Work out the finished part from the listing and answer in its coordinate system (mm). Give positions to 0.01 mm unless a question says otherwise; leave off trailing zeros. Write each loop counter-clockwise with the first axis right and the second up, starting at its lowest first coordinate (ties: lowest second). Pieces come first, ordered by that corner, then holes. Notation, with made-up numbers: (-27.75, 20.25) - (28.25, 20.25) arc R22 ccw to (28.25, 49.25) - close; hole circle Ø6 at (-12.5, -9). An arc over 180 degrees is marked (long way). Write item = value, one per line.
from build123d import *

# Parameters (mm, degrees)
ESBO_O1_R                = 3
RESSALTO_EXTRUS_O1_DEPTH = 5
FILETE1_R                = 6
RESSALTO_EXTRUS_O2_START = 5
RESSALTO_EXTRUS_O2_DEPTH = 5


with BuildPart() as part:
    # Esboço1 → Ressalto-extrusão1 (new body)
    with BuildSketch(Plane.XY):
        Polygon((-8, -8), (-8, 8), (0, 8), (42.879830598, -10.223928004), (37.120169402, -23.776071996), (0, -8), align=None)
        Circle(ESBO_O1_R, mode=Mode.SUBTRACT)
    extrude(amount=RESSALTO_EXTRUS_O1_DEPTH)

    # Filete1
    filete1_edges = [part.edges().sort_by_distance(p)[0] for p in [
        (-8, -8, 2.5),
        (0, -8, 2.5),
        (37.120169402, -23.776071996, 2.5),
        (42.879830598, -10.223928004, 2.5),
        (0, 8, 2.5),
        (-8, 8, 2.5),
    ]]
    fillet(filete1_edges, radius=FILETE1_R)

    # Esboço2 → Ressalto-extrusão2 (add)
    with BuildSketch(Plane.XY.offset(5).offset(RESSALTO_EXTRUS_O2_START)):
        with BuildLine():
            Line((39.467013244, -18.254086485), (40.532986756, -15.745913515))
            ThreePointArc((40.532986756, -15.745913515), (40.575103841, -11.153905468), (37.357845087, -7.877084162))
            ThreePointArc((37.357845087, -7.877084162), (36.552086472, -7.588681558), (35.718304651, -7.395728495))
            ThreePointArc((35.718304651, -7.395728495), (27.413539889, -12.579084175), (31.598183891, -21.429228154))
            ThreePointArc((31.598183891, -21.429228154), (36.190191938, -21.471345238), (39.467013244, -18.254086485))
        make_face()
    extrude(amount=-RESSALTO_EXTRUS_O2_DEPTH)


solid = part.part
1. Find section A-A, the plane z = 1.5. Give the vertices of the cut face in (x, y), then the cut area to 3 significant figures.
Solution:
outline = (-8, -2) arc R6 ccw to (-2, -8) - (-1.22, -8) arc R6 cw to (1.12, -8.48) - (31.6, -21.43) arc R6 ccw to (39.47, -18.25) - (40.53, -15.75) arc R6 ccw to (37.36, -7.88) - (1.12, 7.52) arc R6 ccw to (-1.22, 8) - (-2, 8) arc R6 ccw to (-8, 2) - close; hole circle Ø6 at (0, 0)
area = 709 mm^2
2. For a pull along Y with two mould halves and no side action, classify faces 1 (the cylindrical face through (-3, 0, 2)), 2 (the cylindrical face through (-6.289, 6.196, 2.535)), 3 (the cylindrical face through (-0.041, -8.117, 2.535)), 4 (the flat face through (34, -14, 10)) as pulls with the +Y half, pulls with the -Y half, needs draft (parallel to the pull), parting line crosses it, or undercut.
Solution:
face_1 = undercut
face_2 = pulls with the +Y half
face_3 = pulls with the -Y half
face_4 = needs draft
3. Find section C-C, the plane y = 0. Give the vertices of the cut face in (x, z), then the cut area to 3 significant figures.
Solution:
outline = (-8, 0) - (-3, 0) - (-3, 5) - (-8, 5) - close; (3, 0) - (18.82, 0) - (18.82, 5) - (3, 5) - close
area = 104 mm^2
4. Find section D-D, the plane x = 35. Give the vertices of the cut face in (y, z) (3 decimals), then the cut area to 3 significant figures.
Solution:
outline = (-21.814, 0) - (-6.875, 0) - (-6.875, 5) - (-7.309, 5) - (-7.309, 10) - (-21.814, 10) - close
area = 147 mm^2
5. Straight lines are drawn through the part: line 1 (Z direction, x = 23, y = -16); line 2 (Y direction, x = 0, z = 3.15); line 3 (X direction, y = 2.25, z = 0.75). For each, find the intervals that lie inside material, in ascending order.
Solution:
line_1 = 0 to 5
line_2 = -8.13 to -3, 3 to 7.87
line_3 = -7.99 to -1.98, 1.98 to 13.53
6. Given pin 1 (14.5 mm diameter, centred on x = 15.5, y = -3.5, fed in from +Z); pin 2 (4 mm diameter, centred on x = 8, z = 1, fed in from +Y); pin 3 (2 mm diameter, centred on x = 20.5, z = 2.5, fed in from +Y); pin 4 (5.5 mm diameter, centred on x = 0, y = 0, fed in from -Z), each flat-ended and moving along its own axis, determine where each tip first touches the part or whether it passes through.
Solution:
pin_1 = 5
pin_2 = 5.45
pin_3 = -0.29
pin_4 = through
7. Find section B-B, the plane x = -0.5. Give the vertices of the cut face in (y, z), then the cut area to 3 significant figures.
Solution:
outline = (-8.04, 0) - (-2.96, 0) - (-2.96, 5) - (-8.04, 5) - close; (2.96, 0) - (7.96, 0) - (7.96, 5) - (2.96, 5) - close
area = 50.4 mm^2
